Design review of the part built by this model. Coordinates are the model's own, in mm. Round coordinates to 2 decimals unless told otherwise and drop trailing zeros. Order: outer loops, then holes, each group sorted by start corner. A loop starts at its lowest first (then second) coordinate and runs counter-clockwise, first axis right, second up. Notation, with made-up numbers: M 3,40.25 L 24,40.25 A27 ccw 24,59.25 Z; hole C 71.5,85 d2. An arc over 180 degrees is marked long. Write each question's results on one line, items separated by ' | '. Start each with the question number.
Item 1: Wall thickness on line 1 (Z direction, x = 543, y = -7.25); line 2 (Z direction, x = 101, y = -11.5); line 3 (X direction, y = -7.25, z = 309): over which ranges is each line inside the solid? List them lowest first. Write a range as [from, to].
Item 2: Take a section at B-B, the plane x = 333. Write out the cut boundary in (y, z).
Item 3: Take a section at A-A, the plane y = -12.5. Write out the cut boundary in (x, z), plus the area to 3 significant figures.
Item 4: The part is to be moulded in two halves that separate along Z. For faces 1 (the flat face through (296, -5, 507)), 2 (the flat face through (15, -15, 649)), 3 (the cylindrical face through (590.979, -5.07, 991.445)), 4 (the cylindrical face through (8.555, -5.07, 9.021)), say which applies: +Z half, -Z half, draft (parallel to the pull), parting line (faces both ways), or undercut.
Item 5: Clearance check with a flat-ended pin moving along its axis: pin 1 (4 mm diameter, centred on x = 320, z = 378, fed in from -Y). State where the tip first meets the part, or that it passes through.
Item 6: Take a section at C-C, the plane z = 143. Write out the cut boundary in (x, y), plus the area to 3 significant figures.
```python
from build123d import *

# Parameters (mm, degrees)
F0_W     = 600
F0_H     = 1000
F1_DEPTH = 15
F2_W     = 540
F2_H     = 940
F3_DEPTH = 10
F4_R     = 30
F5_R     = 5
F6_R     = 5


with BuildPart() as f1:
    # F0 (on Front) → F1 (new body)
    with BuildSketch(Plane.XZ):
        with Locations((300, 500)):
            Rectangle(F0_W, F0_H)
    extrude(amount=F1_DEPTH)

    # F2 (on face) → F3 (cut)
    with BuildSketch(Plane.XZ.offset(15)):
        with Locations((300, 500)):
            Rectangle(F2_W, F2_H)
    extrude(amount=-F3_DEPTH, mode=Mode.SUBTRACT)

    # F4
    f4_edges = [f1.edges().sort_by_distance(p)[0] for p in [
        (0, -7.5, 1000),
        (600, -7.5, 1000),
        (600, -7.5, 0),
        (0, -7.5, 0),
    ]]
    fillet(f4_edges, radius=F4_R)

    # F5
    f5_edges = [f1.edges().sort_by_distance(p)[0] for p in [
        (30, -10, 30),
        (570, -10, 30),
        (570, -10, 970),
        (30, -10, 970),
    ]]
    fillet(f5_edges, radius=F5_R)

    # F6
    f6_edges = [f1.edges().sort_by_distance(p)[0] for p in [
        (570, -15, 500),
        (568.535534, -15, 31.464466),
        (568.535534, -15, 968.535534),
        (300, -15, 30),
        (300, -15, 970),
        (31.464466, -15, 31.464466),
        (31.464466, -15, 968.535534),
        (30, -15, 500),
        (0, -15, 500),
        (8.786797, -15, 991.213203),
        (8.786797, -15, 8.786797),
        (300, -15, 1000),
        (300, -15, 0),
        (591.213203, -15, 991.213203),
        (591.213203, -15, 8.786797),
        (600, -15, 500),
    ]]
    fillet(f6_edges, radius=F6_R)


solid = f1.part
```
Results list:
1) line 1: [0, 30], [970, 1000] | line 2: [0.23, 29.77], [970.23, 999.77] | line 3: [0, 30], [570, 600]
2) outline: M -15,5 A5 ccw -10,0 L 0,0 L 0,1000 L -10,1000 A5 ccw -15,995 L -15,975 A5 ccw -10,970 L -5,970 L -5,30 L -10,30 A5 ccw -15,25 Z
3) outline: M 0.67,30 A29.33 ccw 30,0.67 L 570,0.67 A29.33 ccw 599.33,30 L 599.33,970 A29.33 ccw 570,999.33 L 30,999.33 A29.33 ccw 0.67,970 Z; hole M 29.33,35 A5.67 ccw 35,29.33 L 565,29.33 A5.67 ccw 570.67,35 L 570.67,965 A5.67 ccw 565,970.67 L 35,970.67 A5.67 ccw 29.33,965 Z | area: 87,600 mm²
4) face 1: undercut | face 2: draft | face 3: +Z half | face 4: -Z half
5) pin 1: y = -5
6) outline: M 0,-10 A5 ccw 5,-15 L 25,-15 A5 ccw 30,-10 L 30,-5 L 570,-5 L 570,-10 A5 ccw 575,-15 L 595,-15 A5 ccw 600,-10 L 600,0 L 0,0 Z | area: 3,580 mm²
